```python
from build123d import *

# Parameters (mm, degrees)
SKETCH_1_W                = 75
SKETCH_1_H                = 75
EXTRUDE_1_DEPTH           = 10
HOLE_WIZARD_1_D           = 6.6
HOLE_WIZARD_1_DEPTH       = 15
HOLE_WIZARD_1_CBORE_D     = 11
HOLE_WIZARD_1_CBORE_DEPTH = 6.8
HOLE_WIZARD_1_TIP         = 1.982840043
FILLET_1_R                = 3
HOLE_WIZARD_2_D           = 3.4
HOLE_WIZARD_2_CBORE_D     = 6
HOLE_WIZARD_2_CBORE_DEPTH = 3.4


with BuildPart() as part:
    # 草图1 → 凸台-拉伸1 (new body)
    with BuildSketch(Plane.XY):
        Rectangle(SKETCH_1_W, SKETCH_1_H)
    extrude(amount=EXTRUDE_1_DEPTH)

    # 打孔尺寸(%根据)内六角圆柱头螺钉的类型1
    with Locations(Plane(origin=(-25, 25, 10), x_dir=(1, 0, 0), z_dir=(0, 0, 1))):
        with Locations((0, 0), (0, -50), (50, -50), (50, 0)):
            CounterBoreHole(HOLE_WIZARD_1_D / 2, HOLE_WIZARD_1_CBORE_D / 2, HOLE_WIZARD_1_CBORE_DEPTH, depth=HOLE_WIZARD_1_DEPTH)
            with Locations((0, 0, -(HOLE_WIZARD_1_DEPTH + HOLE_WIZARD_1_TIP / 2))):  # 118° drill point
                Cone(0, HOLE_WIZARD_1_D / 2, HOLE_WIZARD_1_TIP, mode=Mode.SUBTRACT)

    # 圆角1
    fillet_1_edges = [part.edges().sort_by_distance(p)[0] for p in [
        (37.5, -37.5, 5),
        (-37.5, -37.5, 5),
        (-37.5, 37.5, 5),
        (37.5, 37.5, 5),
    ]]
    fillet(fillet_1_edges, radius=FILLET_1_R)

    # 打孔尺寸(%根据)内六角圆柱头螺钉的类型2 (through all)
    with Locations(Plane(origin=(0, 0, 0), x_dir=(-1, 0, 0), z_dir=(0, 0, -1))):
        with Locations((13.435028843, -13.435028843), (13.435028843, 13.435028843), (-13.435028843, 13.435028843), (-13.435028843, -13.435028843)):
            CounterBoreHole(HOLE_WIZARD_2_D / 2, HOLE_WIZARD_2_CBORE_D / 2, HOLE_WIZARD_2_CBORE_DEPTH)


solid = part.part
```
Could you check a few things on this model? Use its own coordinates, in mm. A direction names the side the tool comes from. Round coordinates to 2 decimals unless told otherwise and drop trailing zeros. Write each loop counter-clockwise with the first axis right and the second up, starting at its lowest first coordinate (ties: lowest second). Pieces come first, ordered by that corner, then holes. Notation, with made-up numbers: M 0,28 L 43,28 A19 cw 43,59 Z; hole C 3.5,8 d9. An arc over 180 degrees is marked long. Answer in a Markdown table with one row per item. Add a question column.
Q1. If we mould it in two halves opening along X, with no side actions, what happens to faces 4 (the flat face through (-25, -29, 3.2)), 5 (the flat face through (-1, 1, 10)), 6 (the flat face through (-37.5, 0, 5))? For each: +X half, -X half, draft (parallel to the pull), parting line (faces both ways), or undercut.
Q2. Imagine slicing it at A-A (x = 25). Please give me the cut outline in (y, z).
Q3. If I drill on line 1 (Y direction, x = 25, z = 8.5); line 2 (Y direction, x = 25, z = 0.75); line 3 (X direction, y = -12.5, z = 9.75), over which ranges is the centre line in solid material (lowest first)? Write a range as from..to.
Q4. On a 3-axis mill with a long thin cutter (end or side, diameter ignored), from which of +Z, -Z, +X, -X, +Y, -Y can I reach the whole of each face in a straight line? I mean faces 1 (the cylindrical face through (-16.296, 14.336, 1.676)), 2 (the cylindrical face through (-19.754, -23.348, 6.648)), 3 (the cylindrical face through (-14.69, 14.58, 6.75)). Say none if no direction works.
Q5. Will these pins go through, and if not, where does the flat tip stop? pin 1 Ø3.5 at (x, y) = (22.5, -26) entering from +Z; pin 2 Ø5.5 at (x, y) = (-13.44, 13.44) entering from -Z; pin 3 Ø6.5 at (x, y) = (25, 25) entering from -Z.
Q6. Imagine slicing it at C-C (z = 8.5). Give the number of separate pieces and of enclosed holes in the cut face, then the cut area to 3 significant figures.
Values:
| question | item | result |
|---|---|---|
| 1 | face 4 | undercut |
| 1 | face 5 | draft |
| 1 | face 6 | -X half |
| 2 | outline | M -37.5,0 L -28.3,0 L -28.3,3.2 L -30.5,3.2 L -30.5,10 L -37.5,10 Z; M -21.7,0 L 21.7,0 L 21.7,3.2 L 19.5,3.2 L 19.5,10 L -19.5,10 L -19.5,3.2 L -21.7,3.2 Z; M 28.3,0 L 37.5,0 L 37.5,10 L 30.5,10 L 30.5,3.2 L 28.3,3.2 Z |
| 3 | line 1 | -37.5..-30.5, -19.5..19.5, 30.5..37.5 |
| 3 | line 2 | -37.5..-28.3, -21.7..21.7, 28.3..37.5 |
| 3 | line 3 | -37.5..-14.85, -12.02..12.02, 14.85..37.5 |
| 4 | face 1 | -Z |
| 4 | face 2 | +Z |
| 4 | face 3 | +Z, -Z |
| 5 | pin 1 | z = 3.2 |
| 5 | pin 2 | z = 3.4 |
| 5 | pin 3 | through |
| 6 | separate pieces | 1 |
| 6 | enclosed holes | 8 |
| 6 | area | 5,200 mm^2 |
